Work out the finished part from the listing and answer in its coordinate system (mm). Face numbers are marked on the shaded views. Give positions to 0.01 mm unless a question says otherwise; leave off trailing zeros. Loops run counter-clockwise (first coordinate to the right, second up) from the corner with the lowest first, then second, coordinate; pieces in that order, holes last. Notation, with made-up numbers: (50, -20.5) - (66, -20.5) arc R32 cw to (66, 9.5) - close; hole circle Ø4 at (14.5, -16.75). An arc over 180 degrees is marked (long way). Use one line per item in the form item = value. Start each with the question number.
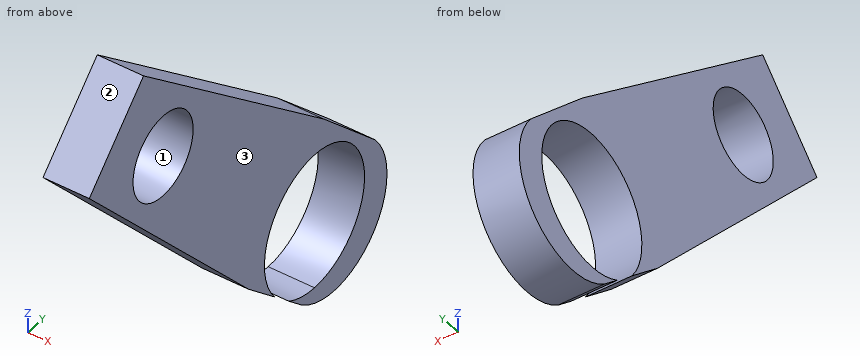
from build123d import *

# Parameters (mm, degrees)
SKETCH1_R           = 13.372971861
BOSS_EXTRUDE1_DEPTH = 14.713458


with BuildPart() as part:
    # Sketch1 → Boss-Extrude1 (new body)
    with BuildSketch(Plane(origin=(0, 0, 0), x_dir=(0, 0, -1), z_dir=(1, 0, 0))):
        with BuildLine():
            Line((-107.077256, 335.05775), (-175.56099, 254.780796))
            Line((-175.56099, 254.780796), (-150.631652, 230.622856))
            Line((-150.631652, 230.622856), (-72.502522, 301.552356))
            Line((-72.502522, 301.552356), (-62.201011559, 313.03589653))
            ThreePointArc((-62.201011559, 313.03589653), (-95.515627855, 340.840078742), (-53.283651357, 330.870306))
            ThreePointArc((-53.283651357, 330.870306), (-54.076724145, 324.9770363), (-56.399514867, 319.50307654))
            Line((-56.399514867, 319.50307654), (-51.143154, 325.36257))
            ThreePointArc((-51.143154, 325.36257), (-53.524433804, 356.502187085), (-84.723478, 357.904288))
            Line((-84.723478, 357.904288), (-107.077256, 335.05775))
        make_face()
        with Locations((-142.853156, 263.47039)):
            Circle(SKETCH1_R, mode=Mode.SUBTRACT)
    extrude(amount=BOSS_EXTRUDE1_DEPTH)


solid = part.part
1) A cutting plane is placed at A-A (z = 74.5). Give the vertices of the cut face in (x, y), plus the area to 3 significant figures.
2) Flat-ended cylindrical pins translate along their axes: pin 1 Ø3 at (x, z) = (2, 125) entering from -Y; pin 2 Ø8 at (x, y) = (12, 300.5) entering from +Z; pin 3 Ø5 at (x, y) = (8, 253) entering from +Z. Find the tip coordinate at first contact, or state that the pin passes through.
3) A cutting plane is placed at D-D (y = 297). Give the vertices of the cut face in (x, z).
4) A cutting plane is placed at B-B (y = 321.5). Give the vertices of the cut face in (x, z).
5) A cutting plane is placed at C-C (x = 9). Give the vertices of the cut face in (y, z).
6) Find the intervals of material crossed by probe 1 along Y at (x, z) = (1.75, 82); probe 2 along Z at (x, y) = (6.75, 326.5); probe 3 along Y at (x, z) = (2.25, 93.5), in increasing order.
7) Determine the mould class of the marked faces 1, 2 and 3 for opening direction Y: released by +Y, released by -Y, zero draft, split by the parting line, or undercut.
Answer sheet:
q1.outline = (0, 299.74) - (14.71, 299.74) - (14.71, 308.6) - (0, 308.6) - close; (0, 353.14) - (14.71, 353.14) - (14.71, 362.69) - (0, 362.69) - close
q1.area = 271 mm²
q2.pin_1 = 252.53
q2.pin_2 = 139.97
q2.pin_3 = 175.56
q3.outline = (0, 77.52) - (14.71, 77.52) - (14.71, 139.54) - (0, 139.54) - close
q4.outline = (0, 54.61) - (14.71, 54.61) - (14.71, 55.35) - (0, 55.35) - close; (0, 95.8) - (14.71, 95.8) - (14.71, 118.64) - (0, 118.64) - close
q5.outline = (230.62, 150.63) - (301.55, 72.5) - (313.04, 62.2) arc R22.29 cw (long way) to (319.5, 56.4) - (325.36, 51.14) arc R23.55 ccw to (357.9, 84.72) - (335.06, 107.08) - (254.78, 175.56) - close; hole circle Ø26.75 at (263.47, 142.85)
q6.probe_1 = 292.93 to 309.52, 352.22 to 359.8
q6.probe_2 = 50.33 to 53.72, 97.44 to 114.38
q6.probe_3 = 282.49 to 317.61, 344.13 to 348.93
q7.face_1 = undercut
q7.face_2 = released by -Y
q7.face_3 = zero draft
